```python
from build123d import *

# Parameters (mm, degrees)
SKETCH_R        = 2.1
SKETCH_R_2      = 1.5
PAD_DEPTH       = 10
POCKET_DEPTH    = 2.5
SKETCH002_R     = 2.1
SKETCH002_R_2   = 1.5
PAD001_DEPTH    = 2
SKETCH003_R     = 3.75
SKETCH003_R_2   = 2.1
POCKET001_DEPTH = 2.5
FILLET_R        = 1
FILLET001_R     = 5
SKETCH004_R     = 1.5
PAD002_DEPTH    = 1


with BuildPart() as part:
    # Sketch → Pad (new body)
    with BuildSketch(Plane.XY):
        with BuildLine():
            Line((-22.5, 10), (22.5, 10))
            Line((22.5, 10), (22.5, -10))
            Line((22.5, -10), (1, -10))
            Line((1, -15), (1, -10))
            ThreePointArc((-11, -15), (-5, -21), (1, -15))
            Line((-11, -15), (-11, -10))
            Line((-22.5, -10), (-11, -10))
            Line((-22.5, -10), (-22.5, 10))
        make_face()
        with Locations((-15, 0)):
            Circle(SKETCH_R, mode=Mode.SUBTRACT)
        with Locations((15, 0)):
            Circle(SKETCH_R, mode=Mode.SUBTRACT)
        with Locations((5, 5)):
            Circle(SKETCH_R_2, mode=Mode.SUBTRACT)
        with Locations((-5, -15)):
            Circle(SKETCH_R_2, mode=Mode.SUBTRACT)
    extrude(amount=PAD_DEPTH)

    # Sketch001 → Pocket (cut)
    with BuildSketch(Plane.XY.offset(10)):
        Polygon((6.587713, 2.25), (8.175426, 5), (6.587713, 7.75), (3.412287, 7.75), (1.824574, 5), (3.412287, 2.25), align=None)
        Polygon((-3.412287, -17.75), (-1.824574, -15), (-3.412287, -12.25), (-6.587713, -12.25), (-8.175426, -15), (-6.587713, -17.75), align=None)
    extrude(amount=-POCKET_DEPTH, mode=Mode.SUBTRACT)

    # Sketch002 → Pad001 (new body)
    with BuildSketch(Plane(origin=(0, 0, 0), x_dir=(1, 0, 0), z_dir=(0, 0, -1))):
        with Locations((5, -5)):
            Circle(SKETCH002_R)
        with Locations((5, -5)):
            Circle(SKETCH002_R_2, mode=Mode.SUBTRACT)
        with Locations((-5, 15)):
            Circle(SKETCH002_R)
        with Locations((-5, 15)):
            Circle(SKETCH002_R_2, mode=Mode.SUBTRACT)
    extrude(amount=PAD001_DEPTH)

    # Sketch003 → Pocket001 (cut)
    with BuildSketch(Plane(origin=(0, 0, 0), x_dir=(1, 0, 0), z_dir=(0, 0, -1))):
        with Locations((15, 0)):
            Circle(SKETCH003_R)
        with Locations((15, 0)):
            Circle(SKETCH003_R_2, mode=Mode.SUBTRACT)
        with Locations((-15, 0)):
            Circle(SKETCH003_R)
        with Locations((-15, 0)):
            Circle(SKETCH003_R_2, mode=Mode.SUBTRACT)
    extrude(amount=-POCKET001_DEPTH, mode=Mode.SUBTRACT)

    # Fillet
    fillet_edges = [part.edges().sort_by_distance(p)[0] for p in [
        (2.9, 5, 0),
        (-7.1, -15, 0),
    ]]
    fillet(fillet_edges, radius=FILLET_R)

    # Fillet001
    fillet001_edges = [part.edges().sort_by_distance(p)[0] for p in [
        (22.5, 10, 5),
        (22.5, -10, 5),
        (-22.5, 10, 5),
        (-22.5, -10, 5),
    ]]
    fillet(fillet001_edges, radius=FILLET001_R)

    # Sketch004 → Pad002 (new body)
    with BuildSketch(Plane.XY.offset(7.5)):
        with Locations((-5, -15)):
            Circle(SKETCH004_R)
        with Locations((5, 5)):
            Circle(SKETCH004_R)
    extrude(amount=-PAD002_DEPTH)


solid = part.part
```
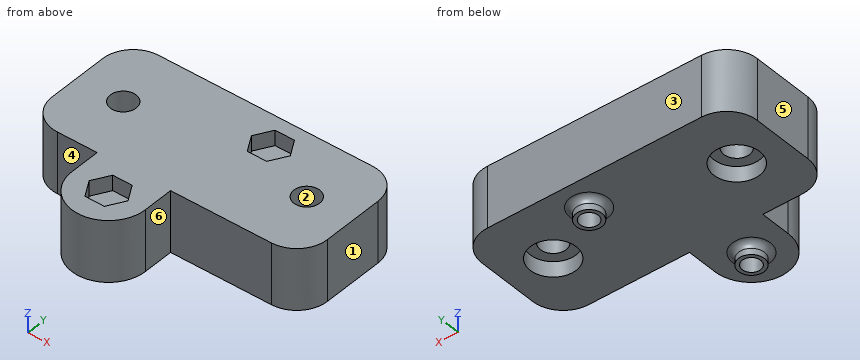
Can you work these out from the model? Positions are in its coordinate system, mm. Face numbers are marked on the shaded views. A direction names the side the tool comes from. Round coordinates to 2 decimals unless told otherwise and drop trailing zeros. Loops run counter-clockwise (first coordinate to the right, second up) from the corner with the lowest first, then second, coordinate; pieces in that order, holes last. Notation, with made-up numbers: M -17,79 L 26,79 A15 ccw 26,107 Z; hole C 32.5,-29 d1. An arc over 180 degrees is marked long. Answer in a Markdown table with one row per item.
1. If we section it at A-A, the plane x = -15: Please give me the cut outline in (y, z).
Established:
| item | result |
|---|---|
| outline | M -10,0 L -3.75,0 L -3.75,2.5 L -2.1,2.5 L -2.1,10 L -10,10 Z; M 2.1,2.5 L 3.75,2.5 L 3.75,0 L 10,0 L 10,10 L 2.1,10 Z |
2. If we section it at C-C, the plane x = 5: Please give me the cut outline in (y, z).
Established:
| item | result |
|---|---|
| outline | M -10,0 L 1.9,0 A1 cw 2.9,-1 L 2.9,-2 L 3.5,-2 L 3.5,6.5 L 6.5,6.5 L 6.5,-2 L 7.1,-2 L 7.1,-1 A1 cw 8.1,0 L 10,0 L 10,10 L 7.75,10 L 7.75,7.5 L 2.25,7.5 L 2.25,10 L -10,10 Z |
3. On a 3-axis mill with a long thin cutter (end or side, diameter ignored), from which of +Z, -Z, +X, -X, +Y, -Y can I reach the whole of each face in a straight line? I mean the marked faces 4, 5 and 6. Say none if no direction works.
Established:
| item | result |
|---|---|
| face 4 | +Z, -Z, -X, -Y |
| face 5 | +Z, -Z, -X, +Y, -Y |
| face 6 | +Z, -Z, +X, -Y |
4. Please list where these lines run through material, in increasing order: line 1 (X direction, y = 0, z = 6); line 2 (X direction, y = -15, z = 3.75); line 3 (Y direction, x = -15, z = 7). Write a range as from..to.
Established:
| item | result |
|---|---|
| line 1 | -22.5..-17.1, -12.9..12.9, 17.1..22.5 |
| line 2 | -11..-6.5, -3.5..1 |
| line 3 | -10..-2.1, 2.1..10 |
5. Thinking about a two-plate mould opening in Y: for the marked faces 1, 2 and 3, which applies, pulls with the +Y half, pulls with the -Y half, needs draft (parallel to the pull), parting line crosses it, or undercut?
Established:
| item | result |
|---|---|
| face 1 | needs draft |
| face 2 | undercut |
| face 3 | pulls with the +Y half |
6. If we section it at D-D, the plane y = -9.5: Please give me the cut outline in (x, z).
Established:
| item | result |
|---|---|
| outline | M -19.68,0 L 19.68,0 L 19.68,10 L -19.68,10 Z |
7. I'm going to push flat-ended pins straight in: pin 1 Ø5.5 at (y, z) = (-11.5, 5) entering from +X; pin 2 Ø8 at (x, y) = (-16.5, -1) entering from -Z; pin 3 Ø3 at (x, z) = (-16, 4) entering from -Y; pin 4 Ø2.5 at (x, y) = (-15, 0) entering from +Z. Where does each tip first touch, or does it pass through?
Established:
| item | result |
|---|---|
| pin 1 | x = 20.81 |
| pin 2 | z = 0 |
| pin 3 | y = -10 |
| pin 4 | through |
8. If we section it at B-B, the plane z = 4: Please give me the cut outline in (x, y).
Established:
| item | result |
|---|---|
| outline | M -22.5,-5 A5 ccw -17.5,-10 L -11,-10 L -11,-15 A6 ccw 1,-15 L 1,-10 L 17.5,-10 A5 ccw 22.5,-5 L 22.5,5 A5 ccw 17.5,10 L -17.5,10 A5 ccw -22.5,5 Z; hole C -15,0 d4.2; hole C -5,-15 d3; hole C 5,5 d3; hole C 15,0 d4.2 |
